The listing builds one solid part. Answer for the finished solid, in the listing's coordinates (mm). A direction names the side the tool comes from. Give positions to 0.01 mm unless a question says otherwise; leave off trailing zeros. Loops run counter-clockwise (first coordinate to the right, second up) from the corner with the lowest first, then second, coordinate; pieces in that order, holes last. Notation, with made-up numbers: (65, 60.25) - (77, 60.25) arc R34 ccw to (77, 96.25) - close; hole circle Ø8 at (24, 65.25). An arc over 180 degrees is marked (long way). Write each question's results on one line, items separated by ' | '.
from build123d import *

# Parameters (mm, degrees)
SKETCH1_R           = 10.5
SKETCH1_R_2         = 0.75
SKETCH1_R_3         = 1.5
BOSS_EXTRUDE1_DEPTH = 2.35
BOSS_EXTRUDE2_START = 2.35
SKETCH1_3_R         = 4.25
SKETCH1_3_R_2       = 2.825
BOSS_EXTRUDE2_DEPTH = 3.65


with BuildPart() as part:
    # Sketch1 → Boss-Extrude1 (new body)
    with BuildSketch(Plane(origin=(0, 0, 0), x_dir=(1, 0, 0), z_dir=(0, 1, 0))):
        Circle(SKETCH1_R)
        with Locations((-7.5, 0)):
            Circle(SKETCH1_R_2, mode=Mode.SUBTRACT)
        with Locations((0, 7.5)):
            Circle(SKETCH1_R_2, mode=Mode.SUBTRACT)
        with Locations((7.5, 0)):
            Circle(SKETCH1_R_2, mode=Mode.SUBTRACT)
        with Locations((0, -7.5)):
            Circle(SKETCH1_R_2, mode=Mode.SUBTRACT)
        Circle(SKETCH1_R_3, mode=Mode.SUBTRACT)
    extrude(amount=BOSS_EXTRUDE1_DEPTH)

    # Sketch1<3> → Boss-Extrude2 (add)
    with BuildSketch(Plane(origin=(0, 0, 0), x_dir=(1, 0, 0), z_dir=(0, 1, 0)).offset(BOSS_EXTRUDE2_START)):
        Circle(SKETCH1_3_R)
        Circle(SKETCH1_3_R_2, mode=Mode.SUBTRACT)
    extrude(amount=BOSS_EXTRUDE2_DEPTH)


solid = part.part
Item 1: Find the intervals of material crossed by line 1 along X through (y, z) = (0.6, 0); line 2 along Y through (x, z) = (4.5, -8.75), in increasing order. Write a range as [from, to].
Values found:
line 1: x = [-10.5, -8.25], [-6.75, -1.5], [1.5, 6.75], [8.25, 10.5] | line 2: y = [0, 2.35]
Item 2: For faces 4 (the face through (1, 6, 3)), 5 (the face through (2.695, 4.149, -0.849)), determine the directions among +Z, -Z, +X, -X, +Y, -Y from which every point of the face is accessible in a straight line to the end or side of a thin tool.
Values found:
face 4: +Z, -Z, +X, -X, +Y | face 5: +Y
Item 3: Flat-ended cylindrical pins translate along their axes: P1, Ø3, axis at x = 3, z = 6, coming from the +Y side; P2, Ø1.5, axis at y = 2, z = 1.5, coming from the -X side; P3, Ø3, axis at y = 2, z = -6.5, coming from the -X side; P4, Ø1.7, axis at x = 0, z = 0, coming from the +Y side. Find the tip coordinate at first contact, or state that the pin passes through.
Values found:
P1: stops at y = 2.35 | P2: stops at x = -10.47 | P3: stops at x = -9.23 | P4: passes through
Item 4: A cutting plane is placed at D-D, the plane z = 7.5. Determine the outline of the cut face in (x, y), plus the area to 3 significant figures.
Values found:
outline: (-7.35, 0) - (-0.75, 0) - (-0.75, 2.35) - (-7.35, 2.35) - close; (0.75, 0) - (7.35, 0) - (7.35, 2.35) - (0.75, 2.35) - close | area: 31.0 mm²
Item 5: For a pull along Z with two mould halves and no side action, classify faces 1 (the face through (2, 0, 0)), 2 (the face through (10, 1.2, -3.2)), 3 (the face through (-1.5, 1.16, -0.07)) as released by +Z, released by -Z, zero draft, split by the parting line, or undercut.
Values found:
face 1: zero draft | face 2: split by the parting line | face 3: undercut
Item 6: A cutting plane is placed at C-C, the plane y = 1.4. Determine the outline of the cut face in (x, z), plus the area to 3 significant figures.
Values found:
outline: circle Ø21 at (0, 0); hole circle Ø1.5 at (-7.5, 0); hole circle Ø3 at (0, 0); hole circle Ø1.5 at (0, -7.5); hole circle Ø1.5 at (0, 7.5); hole circle Ø1.5 at (7.5, 0) | area: 332 mm²
Item 7: A cutting plane is placed at A-A, the plane x = 0. Determine the outline of the cut face in (y, z) (3 decimals), plus the area to 3 significant figures.
Values found:
outline: (0, -10.5) - (2.35, -10.5) - (2.35, -8.25) - (0, -8.25) - close; (0, -6.75) - (2.35, -6.75) - (2.35, -4.25) - (6, -4.25) - (6, -2.825) - (2.35, -2.825) - (2.35, -1.5) - (0, -1.5) - close; (0, 1.5) - (2.35, 1.5) - (2.35, 2.825) - (6, 2.825) - (6, 4.25) - (2.35, 4.25) - (2.35, 6.75) - (0, 6.75) - close; (0, 8.25) - (2.35, 8.25) - (2.35, 10.5) - (0, 10.5) - close | area: 45.7 mm²
Item 8: A cutting plane is placed at B-B, the plane z = 0. Determine the outline of the cut face in (x, y) (3 decimals), plus the area to 3 significant figures.
Values found:
outline: (-10.5, 0) - (-8.25, 0) - (-8.25, 2.35) - (-10.5, 2.35) - close; (-6.75, 0) - (-1.5, 0) - (-1.5, 2.35) - (-2.825, 2.35) - (-2.825, 6) - (-4.25, 6) - (-4.25, 2.35) - (-6.75, 2.35) - close; (1.5, 0) - (6.75, 0) - (6.75, 2.35) - (4.25, 2.35) - (4.25, 6) - (2.825, 6) - (2.825, 2.35) - (1.5, 2.35) - close; (8.25, 0) - (10.5, 0) - (10.5, 2.35) - (8.25, 2.35) - close | area: 45.7 mm²
